Check sheet for the drawn part. Datum: minimum x, y, z corner. Units: mm. Give positions to 0.01 mm unless a question says otherwise; leave off trailing zeros. Loops run counter-clockwise (first coordinate to the right, second up) from the corner with the lowest first, then second, coordinate; pieces in that order, holes last. Notation, with made-up numbers: (-39, 57) - (-28, 57) arc R20 cw to (-28, 81) - close; hole circle Ø11 at (2, -6). An arc over 180 degrees is marked (long way). Answer in a Markdown table with one row per item.
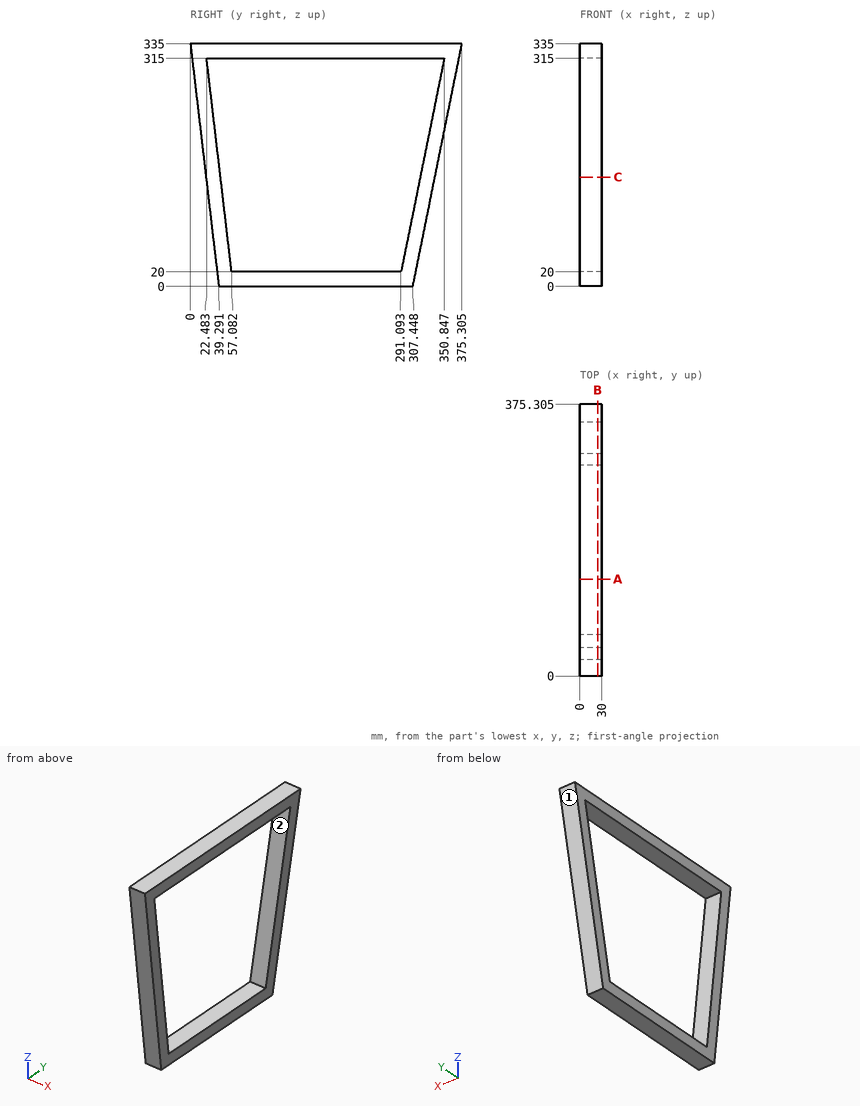
Q1. Sectioned sample at B-B (x = 24.5). Record the cut outline in (y, z) (1 decimal).
Completed:
| item | result |
|---|---|
| outline | (0, 335) - (39.3, 0) - (307.4, 0) - (375.3, 335) - close; hole (22.5, 315) - (57.1, 20) - (291.1, 20) - (350.8, 315) - close |
Q2. Sectioned sample at C-C (z = 151). Record the cut outline in (x, y), and give its area (3 significant figures).
Completed:
| item | result |
|---|---|
| outline | (0, 21.58) - (30, 21.58) - (30, 41.72) - (0, 41.72) - close; (0, 317.63) - (30, 317.63) - (30, 338.03) - (0, 338.03) - close |
| area | 1,220 mm^2 |
Q3. Thickness scan on line 1 (Z direction, x = 13.75, y = 212); line 2 (Y direction, x = 4.25, z = 43.5) (1 decimal); line 3 (Y direction, x = 14.25, z = 46) (1 decimal). Record the ranges inside material, lowest first.
Completed:
| item | result |
|---|---|
| line 1 | 0 to 20, 315 to 335 |
| line 2 | 34.2 to 54.3, 295.9 to 316.3 |
| line 3 | 33.9 to 54, 296.4 to 316.8 |
Q4. Sectioned sample at A-A (y = 134). Record the cut outline in (x, z).
Completed:
| item | result |
|---|---|
| outline | (0, 0) - (30, 0) - (30, 20) - (0, 20) - close; (0, 315) - (30, 315) - (30, 335) - (0, 335) - close |
Q5. Draft check along Y on the marked faces 1 and 2. Enter one of: +Y half, -Y half, draft (parallel to the pull), parting line (faces both ways), or undercut.
Completed:
| item | result |
|---|---|
| face 1 | +Y half |
| face 2 | undercut |
